Verification items for the finished model (mm, model axes). A direction names the side the tool comes from. Round coordinates to 2 decimals unless told otherwise and drop trailing zeros. Write each loop counter-clockwise with the first axis right and the second up, starting at its lowest first coordinate (ties: lowest second). Pieces come first, ordered by that corner, then holes.
from build123d import *

# Parameters (mm, degrees)
F0_W     = 103.471577
F0_H     = 135.355264
F0_W_2   = 83.017897
F0_H_2   = 117.608685
F1_DEPTH = 127
F0_W_3   = 57.149997
F0_H_3   = 101.366054
F2_DEPTH = 76.2


with BuildPart() as f1:
    # F0 (on Front) → F1 (new body)
    with BuildSketch(Plane.XZ):
        with Locations((0.150393, -0.751972)):
            Rectangle(F0_W, F0_H)
        with Locations((2.55671, -0.30079)):
            Rectangle(F0_W_2, F0_H_2, mode=Mode.SUBTRACT)
    extrude(amount=F1_DEPTH)

    # F0 (on Front) → F2 (join)
    with BuildSketch(Plane.XZ):
        with Locations((2.55671, -0.30079)):
            Rectangle(F0_W_2, F0_H_2)
        with Locations((3.158288, 1.50395)):
            Rectangle(F0_W_3, F0_H_3, mode=Mode.SUBTRACT)
    extrude(amount=F2_DEPTH)


solid = f1.part
Q1. Tool access check on faces 4 (the flat face through (-35, 0, 0)), 5 (the flat face through (3, -38, 52.187)), 6 (the flat face through (2, -101, -59.105)). Record the directions out of +Z, -Z, +X, -X, +Y, -Y that give a thin tool (end or side, any length) a straight path to the whole face; none if there is none.
Recorded:
face 4: +Z, -Z, +X, -X, +Y
face 5: +Y, -Y
face 6: -Y
Q2. Sectioned sample at B-B (x = 29.5). Enter the section's corners in (y, z), plus the area to 3 significant figures.
Recorded:
outline: (-127, -68.43) - (0, -68.43) - (0, -49.18) - (-76.2, -49.18) - (-76.2, -59.11) - (-127, -59.11) - close; (-127, 58.5) - (-76.2, 58.5) - (-76.2, 52.19) - (0, 52.19) - (0, 66.93) - (-127, 66.93) - close
area: 3,490 mm2
Q3. Material ranges on line 1 along X through (y, z) = (-116, 53); line 2 along X through (y, z) = (-37.5, -9); line 3 along Z through (x, y) = (-14.5, -104.5), recorded low to high.
Recorded:
line 1: x = -51.59 to -38.95, 44.07 to 51.89
line 2: x = -51.59 to -25.42, 31.73 to 51.89
line 3: z = -68.43 to -59.11, 58.5 to 66.93
Q4. Sectioned sample at D-D (y = -108.5). Enter the section's corners in (x, z), plus the area to 3 significant figures.
Recorded:
outline: (-51.59, -68.43) - (51.89, -68.43) - (51.89, 66.93) - (-51.59, 66.93) - close; hole (-38.95, -59.11) - (44.07, -59.11) - (44.07, 58.5) - (-38.95, 58.5) - close
area: 4,240 mm2
Q5. Sectioned sample at C-C (y = -38.5). Enter the section's corners in (x, z), plus the area to 3 significant figures.
Recorded:
outline: (-51.59, -68.43) - (51.89, -68.43) - (51.89, 66.93) - (-51.59, 66.93) - close; hole (-25.42, -49.18) - (31.73, -49.18) - (31.73, 52.19) - (-25.42, 52.19) - close
area: 8,210 mm2
Q6. Release check for a two-part mould opening along Z. For faces 1 (the flat face through (51.886, -63, -2)), 2 (the flat face through (-26, -76.2, 1)), 3 (the flat face through (-1, -63, -68.43)) record: released by +Z, released by -Z, zero draft, split by the parting line, or undercut.
Recorded:
face 1: zero draft
face 2: undercut
face 3: released by -Z
Q7. Sectioned sample at A-A (z = -5). Enter the section's corners in (x, y).
Recorded:
outline: (-51.59, -127) - (-38.95, -127) - (-38.95, -76.2) - (-25.42, -76.2) - (-25.42, 0) - (-51.59, 0) - close; (31.73, -76.2) - (44.07, -76.2) - (44.07, -127) - (51.89, -127) - (51.89, 0) - (31.73, 0) - close
